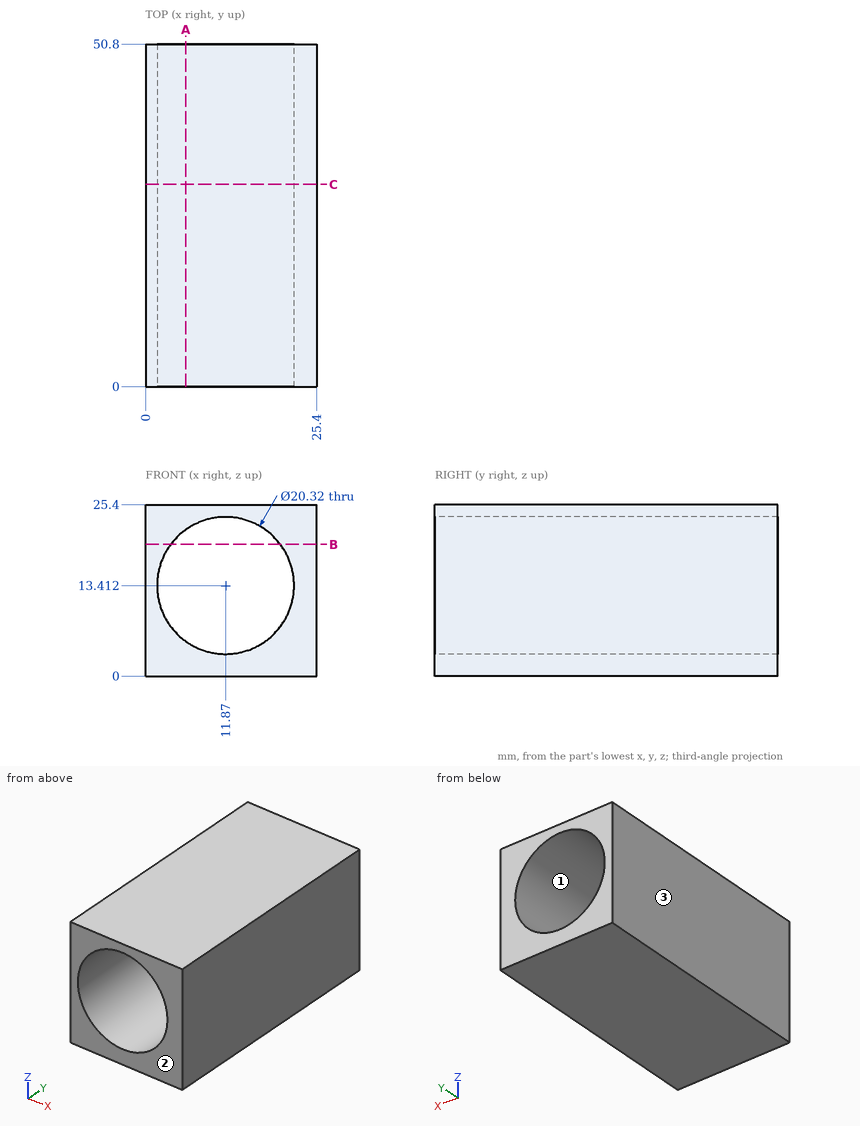
Geometry check sheet. Reference: drawing and pictorial views, mm from the part's lowest x, y, z. Give positions to 0.01 mm unless a question says otherwise; leave off trailing zeros. Loops run counter-clockwise (first coordinate to the right, second up) from the corner with the lowest first, then second, coordinate; pieces in that order, holes last. Notation, with made-up numbers: (62, -28.75) -> (104, -28.75) arc R18 ccw to (104, -23.75) -> close; hole circle Ø1 at (-20.5, 85). An arc over 180 degrees is marked (long way). Answer in a Markdown table with one row per item. Add a question column.
1) Cross-section at A-A on x = 6. Record the boundary of the cut face in (y, z) (1 decimal).
2) Cross-section at C-C on y = 30. Record the boundary of the cut face in (x, z).
3) Draft check along X on the marked faces 1, 2 and 3. Enter one of: pulls with the +X half, pulls with the -X half, needs draft (parallel to the pull), parting line crosses it, or undercut.
4) Cross-section at B-B on z = 19.5. Record the boundary of the cut face in (x, y) (1 decimal), and give its area (3 significant figures).
5) Material ranges on probe 1 along Z at (x, y) = (11.5, 33) (1 decimal); probe 2 along X at (y, z) = (43, 18.75) (1 decimal); probe 3 along Z at (x, y) = (14.5, 30) (1 decimal), recorded low to high. Write a range as from..to.
Outcome:
| question | item | result |
|---|---|---|
| 1 | outline | (0, 0) -> (50.8, 0) -> (50.8, 5.1) -> (0, 5.1) -> close; (0, 21.7) -> (50.8, 21.7) -> (50.8, 25.4) -> (0, 25.4) -> close |
| 2 | outline | (0, 0) -> (25.4, 0) -> (25.4, 25.4) -> (0, 25.4) -> close; hole circle Ø20.32 at (11.87, 13.41) |
| 3 | face 1 | undercut |
| 3 | face 2 | needs draft |
| 3 | face 3 | pulls with the -X half |
| 4 | outline | (0, 0) -> (3.7, 0) -> (3.7, 50.8) -> (0, 50.8) -> close; (20, 0) -> (25.4, 0) -> (25.4, 50.8) -> (20, 50.8) -> close |
| 4 | area | 464 mm^2 |
| 5 | probe 1 | z = 0..3.3, 23.6..25.4 |
| 5 | probe 2 | x = 0..3.2, 20.5..25.4 |
| 5 | probe 3 | z = 0..3.6, 23.2..25.4 |
